Part model, mm, in its own coordinate system. Face numbers are marked on the shaded views. A direction names the side the tool comes from. Round coordinates to 2 decimals unless told otherwise and drop trailing zeros. Loops run counter-clockwise (first coordinate to the right, second up) from the corner with the lowest first, then second, coordinate; pieces in that order, holes last.
(1) Cut at C-C on x = -66. List the corners of the cut face in (y, z), then the cut area to 3 significant figures.
(2) Mould opens along Z. For the marked faces 4, 5 and 6 say: +Z half, -Z half, draft (parallel to the pull), parting line (faces both ways), or undercut.
(3) Tool access for the marked faces 1, 2 and 3: list every direction of +Z, -Z, +X, -X, +Y, -Y with a clear straight run to the whole face (end or side of a thin tool).
(4) Cut at A-A on z = -12.7. List the corners of the cut face in (x, y).
(5) Cut at B-B on x = 44.45. List the corners of the cut face in (y, z).
(6) Flat gauge pins, fed straight in: pin 1 (10 mm diameter, centred on x = -73.5, y = -32.5, fed in from +Z); pin 2 (1 mm diameter, centred on x = -5, z = -13, fed in from -Y); pin 3 (19 mm diameter, centred on x = -9, y = -60.5, fed in from -Z). Where does each tip first touch, or does it go through?
(7) Cut at D-D on z = 16.5. List the corners of the cut face in (x, y).
(8) Probe probe 1 along X at (y, z) = (-6, -12); probe 2 along Z at (x, y) = (44.45, -8.5); probe 3 along Z at (x, y) = (-47, -53.5). List the from-to ranges inside material, lowest first.
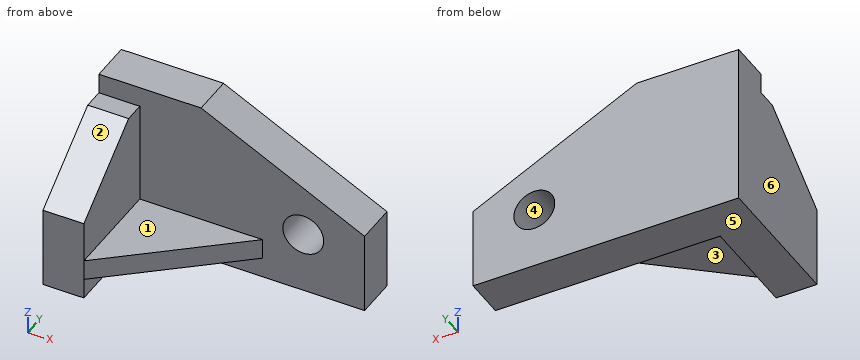
from build123d import *

# Parameters (mm, degrees)
F0_W     = 76.2
F0_H     = 12.7
F0_W_2   = 25.4
F0_H_2   = 38.1
F1_DEPTH = 88.9
F0_R     = 12.7
F2_DEPTH = 25.4
F4_DEPTH = 25.4
F6_DEPTH = 25.4


with BuildPart() as f1:
    # F0 (on Front) → F1 (new body)
    with BuildSketch(Plane.XZ):
        with Locations((-19.05, -31.75)):
            Rectangle(F0_W, F0_H)
        Polygon((-82.55, -50.8), (-57.15, -50.8), (-57.15, -38.1), (-57.15, -25.4), (-57.15, 0), (-82.55, 0), align=None)
        with Locations((-69.85, 19.05)):
            Rectangle(F0_W_2, F0_H_2)
    extrude(amount=F1_DEPTH)

    # F0 (on Front) → F2 (join)
    with BuildSketch(Plane.XZ):
        Polygon((-82.55, -50.8), (-57.15, -50.8), (-57.15, -38.1), (-57.15, -25.4), (-57.15, 0), (-82.55, 0), align=None)
        Polygon((82.55, 0), (-19.05, 50.8), (-82.55, 50.8), (-82.55, 38.1), (-57.15, 38.1), (-57.15, 0), (-57.15, -25.4), (19.05, -25.4), (19.05, -38.1), (-57.15, -38.1), (-57.15, -50.8), (82.55, -50.8), align=None)
        with Locations((44.45, -12.7)):
            Circle(F0_R, mode=Mode.SUBTRACT)
    extrude(amount=F2_DEPTH)

    # F3 (on face) → F4 (cut)
    with BuildSketch(Plane.YZ.offset(-57.15)):
        Polygon((-88.9, 0), (-38.1, 38.1), (-88.9, 38.1), align=None)
    extrude(amount=-F4_DEPTH, mode=Mode.SUBTRACT)

    # F5 (on face) → F6 (cut)
    with BuildSketch(Plane.XY.offset(-25.4)):
        Polygon((19.05, -88.9), (19.05, -25.4), (-57.15, -88.9), align=None)
    extrude(amount=-F6_DEPTH, mode=Mode.SUBTRACT)


solid = f1.part
Final values:
1. outline: (-88.9, -50.8) - (0, -50.8) - (0, 50.8) - (-25.4, 50.8) - (-25.4, 38.1) - (-38.1, 38.1) - (-88.9, 0) - close
1. area: 7,260 mm2
2. face 4: undercut
2. face 5: -Z half
2. face 6: draft
3. face 1: +Z, +X, -Y
3. face 2: +Z, +X, -X, -Y
3. face 3: -Z, +X, -Y
4. outline: (-82.55, -88.9) - (-57.15, -88.9) - (-57.15, -25.4) - (31.75, -25.4) - (31.75, 0) - (-82.55, 0) - close; (57.15, -25.4) - (82.55, -25.4) - (82.55, 0) - (57.15, 0) - close
5. outline: (-25.4, -50.8) - (0, -50.8) - (0, -25.4) - (-25.4, -25.4) - close; (-25.4, 0) - (0, 0) - (0, 19.05) - (-25.4, 19.05) - close
6. pin 1: stops at z = 38.1
6. pin 2: stops at y = -25.4
6. pin 3: stops at z = -38.1
7. outline: (-82.55, -66.9) - (-57.15, -66.9) - (-57.15, -25.4) - (49.55, -25.4) - (49.55, 0) - (-82.55, 0) - close
8. probe 1: x = -82.55 to 31.77, 57.13 to 82.55
8. probe 2: z = -50.8 to -25.4, 0 to 19.05
8. probe 3: z = -38.1 to -25.4
